Could you check a few things on this model? Use its own coordinates, in mm. Coordinates: 2 decimals unless noted, no trailing zeros. Write each loop counter-clockwise with the first axis right and the second up, starting at its lowest first coordinate (ties: lowest second). Pieces come first, ordered by that corner, then holes. Notation, with made-up numbers: M 36,43 L 85,43 A26 cw 85,82 Z; hole C -22.5,-24.5 d1. An arc over 180 degrees is marked long. Write item = value, one per line.
```python
from build123d import *

# Parameters (mm, degrees)
F1_R      = 12.7
F2_DEPTH  = 268.2875
F6_W      = 114.097729
F6_H      = 88.5094
F7_DEPTH  = 25.4
F11_W     = 145.65833
F11_H     = 82.475946
F12_DEPTH = 25.4


with BuildPart() as f2:
    # F1 (on face) → F2 (new body)
    with BuildSketch(Plane.XZ):
        Circle(F1_R)
    extrude(amount=F2_DEPTH)

    # F6 (on face) → F7 (cut)
    with BuildSketch(Plane(origin=(92.994083, -224.507577, 0), x_dir=(-0.92388, -0.382683, 0), z_dir=(-0.382683, 0.92388, 0))):
        with Locations((118.185877, 2.949333)):
            Rectangle(F6_W, F6_H)
    extrude(amount=-F7_DEPTH, mode=Mode.SUBTRACT)

    # F11 (on face) → F12 (cut)
    with BuildSketch(Plane(origin=(-1.859872, -4.490128, 0), x_dir=(-0.92388, 0.382683, 0), z_dir=(0.382683, 0.92388, 0))):
        Rectangle(F11_W, F11_H)
    extrude(amount=F12_DEPTH, mode=Mode.SUBTRACT)


solid = f2.part
```
Item 1: Imagine slicing it at C-C (x = -1). Write out the boundary of the cut face in (y, z).
Numbers:
outline = M -263.44,-12.66 L -4.85,-12.66 L -4.85,12.66 L -263.44,12.66 Z
Item 2: Imagine slicing it at B-B (z = 0). Write out the boundary of the cut face in (x, y), and give its area (3 significant figures).
Numbers:
outline = M -12.7,-268.29 L 12.7,-257.77 L 12.7,-10.52 L -12.7,0 Z
area = 6,550 mm²
Item 3: I'm going to push flat-ended pins straight in: P1, Ø12, axis at x = 1, z = 1, coming from the +Y side; P2, Ø3, axis at x = -5.5, y = -95.5, coming from the -Z side; P3, Ø5, axis at x = 8.5, z = 6, coming from the +Y side. Where does each tip first touch, or does it pass through?
Numbers:
P1 = -3.19
P2 = -12.05
P3 = -7.75
Item 4: Imagine slicing it at A-A (y = -222). Write out the boundary of the cut face in (x, z), and give its area (3 significant figures).
Numbers:
outline = C 0,0 d25.4
area = 507 mm²
Item 5: If I drill on line 1 along X through (y, z) = (-15.5, 1); line 2 along Z through (x, y) = (-0.25, -30); line 3 along Z through (x, y) = (-1.25, -243), over which ranges is the centre line in solid material (lowest first)?
Numbers:
line_1 = -12.66 to 12.66
line_2 = -12.7 to 12.7
line_3 = -12.64 to 12.64
